```python
from build123d import *

# Parameters (mm, degrees)
SKETCH1_R               = 1.75
BOSS_EXTRUDE3_DEPTH     = 3
SKETCH4_W               = 38.009499712
SKETCH4_H               = 2.5
CUT_EXTRUDE7_DEPTH      = 29.268853886
SKETCH7_W               = 36
SKETCH7_H               = 1
CUT_EXTRUDE8_DEPTH      = 47.877632193
SKETCH9_W               = 39.982004405
SKETCH9_H               = 3.901650926
SKETCH9_W_2             = 38.509499712
SKETCH9_H_2             = 2.8
SKETCH9_W_3             = 37.982004405
SKETCH9_H_3             = 0.55
CUT_EXTRUDE9_DEPTH      = 10
SKETCH10_W              = 40
SKETCH10_H              = 4
SKETCH10_W_2            = 39.982004405
SKETCH10_H_2            = 3.901650926
CUT_EXTRUDE11_DEPTH     = 29.180278565
SKETCH11_W              = 20
SKETCH11_H              = 3.116121774
CUT_EXTRUDE12_DEPTH     = 10
SKETCH12_W              = 2
SKETCH12_H              = 8.5
CUT_EXTRUDE15_DEPTH     = 10
CROQUIS1_W              = 24
CROQUIS1_H              = 4
SALIENTE_EXTRUIR1_DEPTH = 2
CROQUIS2_W              = 40
CROQUIS2_H              = 4
SALIENTE_EXTRUIR2_DEPTH = 4
CORTAR_EXTRUIR2_DEPTH   = 4
SKETCH3_W               = 9
SKETCH3_H               = 3.998143652
CORTAR_EXTRUIR5_DEPTH   = 4


with BuildPart() as part:
    # Sketch1 → Boss-Extrude3 (new body)
    # profile 1 of 2: a face of its own
    with BuildSketch(Plane(origin=(0, 0, 0), x_dir=(1, 0, 0), z_dir=(0, 1, 0))):
        Polygon((-21.59, 18), (-21.59, 0), (0, 0), (21.59, 0), (21.59, 18), (18.04585781, 18), (10.04585781, 18), (10.04585781, 12.616121774), (-9.95414219, 12.616121774), (-9.95414219, 18), (-17.95414219, 18), align=None)
        with Locations(Location((-15, 15, 0), (0, 0, 270))):
            Circle(SKETCH1_R, mode=Mode.SUBTRACT)
        Polygon((18.504745017, 6.25), (0, 6.25), (-18.5, 6.25), (-19.004539265, 6.25), (-19.004539265, 8.75), (-18.5, 8.75), (0.002372509, 8.75), (18.504745017, 8.75), (19.004960447, 8.75), (19.004960447, 6.25), align=None, mode=Mode.SUBTRACT)
        with Locations(Location((15, 15, 0), (0, 0, 270))):
            Circle(SKETCH1_R, mode=Mode.SUBTRACT)
    # profile 2 of 2: a face of its own
    with BuildSketch(Plane(origin=(0, 0, 0), x_dir=(1, 0, 0), z_dir=(0, 1, 0))):
        Polygon((0, 0), (-21.59, 0), (-21.59, -18), (-17.95414219, -18), (-9.95414219, -18), (-9.95414219, -12.616121774), (10.04585781, -12.616121774), (10.04585781, -18), (18.04585781, -18), (21.59, -18), (21.59, 0), align=None)
        with Locations(Location((-15, -15, 0), (0, 0, 270))):
            Circle(SKETCH1_R, mode=Mode.SUBTRACT)
        with Locations(Location((15, -15, 0), (0, 0, 270))):
            Circle(SKETCH1_R, mode=Mode.SUBTRACT)
        Polygon((18.504745017, -6.25), (19.004960447, -6.25), (19.004960447, -8.75), (18.504745017, -8.75), (-18.5, -8.75), (-19.004539265, -8.75), (-19.004539265, -6.25), (-18.5, -6.25), align=None, mode=Mode.SUBTRACT)
    extrude(amount=BOSS_EXTRUDE3_DEPTH)

    # Sketch4 → Cut-Extrude7 (cut, through all)
    # profile 1 of 3: a face of its own
    with BuildSketch(Plane(origin=(0, 3, 0), x_dir=(1, 0, 0), z_dir=(0, 1, 0))):
        Polygon((19.004960447, 6.1), (19.254960447, 6.1), (19.254960447, 8.882786661), (19.254960447, 8.9), (19.004960447, 8.9), (-19.004539265, 8.9), (-19.254539265, 8.9), (-19.254539265, 6.1), (-19.004539265, 6.1), align=None)
        with Locations((0.000210591, 7.5)):
            Rectangle(SKETCH4_W, SKETCH4_H, mode=Mode.SUBTRACT)
    # profile 2 of 3: a face of its own
    with BuildSketch(Plane(origin=(0, 3, 0), x_dir=(1, 0, 0), z_dir=(0, 1, 0))):
        with Locations((0.000210591, 7.5)):
            Rectangle(SKETCH4_W, SKETCH4_H)
    # profile 3 of 3: a face of its own
    with BuildSketch(Plane(origin=(0, 3, 0), x_dir=(1, 0, 0), z_dir=(0, 1, 0))):
        Polygon((-19.254539265, -6.1), (-19.254539265, -8.9), (-19.004539265, -8.9), (19.004960447, -8.9), (19.254960447, -8.9), (19.254960447, -6.1), (19.004960447, -6.1), (-19.004539265, -6.1), align=None)
        with Locations((0.000210591, -7.5)):
            Rectangle(SKETCH4_W, SKETCH4_H, mode=Mode.SUBTRACT)
    extrude(amount=-CUT_EXTRUDE7_DEPTH, mode=Mode.SUBTRACT)

    # Sketch7 → Cut-Extrude8 (cut, through all)
    with BuildSketch(Plane(origin=(21.59, 0, 0), x_dir=(0, 0, -1), z_dir=(1, 0, 0))):
        with Locations((0, 0.5)):
            Rectangle(SKETCH7_W, SKETCH7_H)
    extrude(amount=-CUT_EXTRUDE8_DEPTH, mode=Mode.SUBTRACT)

    # Sketch9 → Cut-Extrude9 (cut)
    # profile 1 of 4: a face of its own
    with BuildSketch(Plane(origin=(0, 3, 0), x_dir=(1, 0, 0), z_dir=(0, 1, 0))):
        with Locations((0.000210592, 7.5)):
            Rectangle(SKETCH9_W, SKETCH9_H)
        with Locations((0.000210591, 7.5)):
            Rectangle(SKETCH9_W_2, SKETCH9_H_2, mode=Mode.SUBTRACT)
    # profile 2 of 4: a face of its own
    with BuildSketch(Plane(origin=(0, 3, 0), x_dir=(1, 0, 0), z_dir=(0, 1, 0))):
        with Locations((0.000210592, -7.5)):
            Rectangle(SKETCH9_W, SKETCH9_H)
        Polygon((-19.254539265, -8.9), (-19.254539265, -6.1), (-18.990791611, -6.1), (-18.990791611, -5.55), (18.991212794, -5.55), (18.991212794, -6.1), (19.254960447, -6.1), (19.254960447, -8.9), (18.991212794, -8.9), (18.991212794, -9.45), (-18.990791611, -9.45), (-18.990791611, -8.9), align=None, mode=Mode.SUBTRACT)
    # profile 3 of 4: a face of its own
    with BuildSketch(Plane(origin=(0, 3, 0), x_dir=(1, 0, 0), z_dir=(0, 1, 0))):
        with Locations((0.000210592, -5.825)):
            Rectangle(SKETCH9_W_3, SKETCH9_H_3)
    # profile 4 of 4: a face of its own
    with BuildSketch(Plane(origin=(0, 3, 0), x_dir=(1, 0, 0), z_dir=(0, 1, 0))):
        with Locations((0.000210592, -9.175)):
            Rectangle(SKETCH9_W_3, SKETCH9_H_3)
    extrude(amount=-CUT_EXTRUDE9_DEPTH, mode=Mode.SUBTRACT)

    # Sketch10 → Cut-Extrude11 (cut, through all)
    # profile 1 of 3: a face of its own
    with BuildSketch(Plane(origin=(0, 3, 0), x_dir=(1, 0, 0), z_dir=(0, 1, 0))):
        with Locations((0.000210591, -7.5)):
            Rectangle(SKETCH10_W, SKETCH10_H)
        with Locations((0.000210592, -7.5)):
            Rectangle(SKETCH10_W_2, SKETCH10_H_2, mode=Mode.SUBTRACT)
    # profile 2 of 3: a face of its own
    with BuildSketch(Plane(origin=(0, 3, 0), x_dir=(1, 0, 0), z_dir=(0, 1, 0))):
        with Locations((0.000210591, 7.5)):
            Rectangle(SKETCH10_W, SKETCH10_H)
        with Locations((0.000210592, 7.5)):
            Rectangle(SKETCH10_W_2, SKETCH10_H_2, mode=Mode.SUBTRACT)
    # profile 3 of 3: a face of its own
    with BuildSketch(Plane(origin=(0, 3, 0), x_dir=(1, 0, 0), z_dir=(0, 1, 0))):
        with Locations((0.000210592, 7.5)):
            Rectangle(SKETCH10_W_2, SKETCH10_H_2)
    extrude(amount=-CUT_EXTRUDE11_DEPTH, mode=Mode.SUBTRACT)

    # Sketch11 → Cut-Extrude12 (cut)
    with BuildSketch(Plane(origin=(0, 3, 0), x_dir=(1, 0, 0), z_dir=(0, 1, 0))):
        with Locations((0.04585781, -11.058060887)):
            Rectangle(SKETCH11_W, SKETCH11_H)
        with Locations((0.04585781, 11.058060887)):
            Rectangle(SKETCH11_W, SKETCH11_H)
    extrude(amount=-CUT_EXTRUDE12_DEPTH, mode=Mode.SUBTRACT)

    # Sketch12 → Cut-Extrude15 (cut)
    with BuildSketch(Plane(origin=(0, 3, 0), x_dir=(1, 0, 0), z_dir=(0, 1, 0))):
        with Locations((-10.95414219, -13.75)):
            Rectangle(SKETCH12_W, SKETCH12_H)
        with Locations((-10.95414219, 13.75)):
            Rectangle(SKETCH12_W, SKETCH12_H)
        with Locations((11.04585781, 13.75)):
            Rectangle(SKETCH12_W, SKETCH12_H)
        Polygon((10.04585781, -9.65592739), (10.04585781, -18), (12.04585781, -18), (12.04585781, -9.65592739), (12.04585781, -9.5), (10.04585781, -9.5), align=None)
    extrude(amount=-CUT_EXTRUDE15_DEPTH, mode=Mode.SUBTRACT)

    # Croquis1 → Saliente-Extruir1 (add)
    with BuildSketch(Plane(origin=(0, 3, 0), x_dir=(1, 0, 0), z_dir=(0, 1, 0))):
        with Locations((0.04585781, -11.5)):
            Rectangle(CROQUIS1_W, CROQUIS1_H)
        with Locations((0.04585781, 11.5)):
            Rectangle(CROQUIS1_W, CROQUIS1_H)
    extrude(amount=-SALIENTE_EXTRUIR1_DEPTH)

    # Croquis2 → Saliente-Extruir2 (add)
    with BuildSketch(Plane(origin=(0, 3, 0), x_dir=(1, 0, 0), z_dir=(0, 1, 0))):
        Polygon((21.59, 9.27), (21.59, 12.25), (-21.59, 12.25), (-21.59, 9.27), (-21.59, -9.27), (-21.59, -12.25), (21.59, -12.25), (21.59, -9.27), align=None)
        with Locations((0.000210591, -7.5)):
            Rectangle(CROQUIS2_W, CROQUIS2_H, mode=Mode.SUBTRACT)
        with Locations((0.000210591, 7.5)):
            Rectangle(CROQUIS2_W, CROQUIS2_H, mode=Mode.SUBTRACT)
    extrude(amount=SALIENTE_EXTRUIR2_DEPTH)

    # Croquis4 → Cortar-Extruir2 (cut)
    with BuildSketch(Plane.XZ.offset(-1)):
        Polygon((-21.59, -9.5), (-21.59, 9.5), (-19.999789409, 9.5), (-19.999789409, 5.5), (20.000210591, 5.5), (20.000210591, 9.5), (21.59, 9.5), (21.59, -9.5), (20.000210591, -9.5), (20.000210591, -5.5), (-19.999789409, -5.5), (-19.999789409, -9.5), align=None)
    extrude(amount=-CORTAR_EXTRUIR2_DEPTH, mode=Mode.SUBTRACT)

    # Sketch3 → Cortar-Extruir5 (cut)
    with BuildSketch(Plane(origin=(0, 3, 0), x_dir=(1, 0, 0), z_dir=(0, 1, 0))):
        Polygon((-1.911780511, -2), (-1.911780511, 0), (-3.40804733, 0), (-3.911780511, 0), (-3.911780511, -0.084828213), (-3.911780511, -2), align=None)
        Polygon((-3.40804733, 0), (-1.911780511, 0), (-1.911780511, 2), (-3.911780511, 2), (-3.911780511, 0), align=None)
        Polygon((12.59, 0.000697543), (12.59, 0), (21.59, 0), (21.59, 3.999538738), (12.59, 3.999538738), align=None)
        with Locations((17.09, -1.999071826)):
            Rectangle(SKETCH3_W, SKETCH3_H)
        Polygon((-16.59, -3.75), (-16.59, 0), (-16.59, 3.75), (-21.59, 3.75), (-21.59, 0), (-21.59, -3.75), align=None)
    extrude(amount=CORTAR_EXTRUIR5_DEPTH, mode=Mode.SUBTRACT)


solid = part.part
```
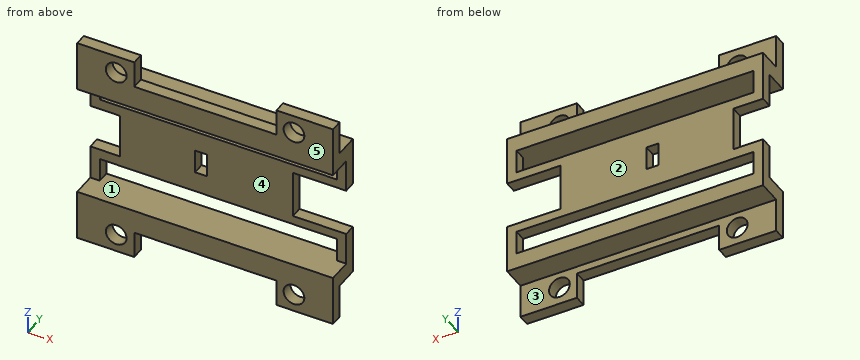
The listing builds one solid part. Answer for the finished solid, in the listing's coordinates (mm). Face numbers are marked on the shaded views. A direction names the side the tool comes from. Give positions to 0.01 mm unless a question says otherwise; leave off trailing zeros. Order: outer loops, then holes, each group sorted by start corner. A loop starts at its lowest first (then second) coordinate and runs counter-clockwise, first axis right, second up.
1) For the marked faces 3, 4 and 5, determine the directions among +Z, -Z, +X, -X, +Y, -Y from which every point of the face is accessible in a straight line to the end or side of a thin tool.
Reported:
face 3: -Z, +X, -X, +Y
face 4: +X, -X, -Y
face 5: +Z, -Z, +X, -X, -Y
2) Determine the mould class of the marked faces 1 and 2 for opening direction X: pulls with the +X half, pulls with the -X half, needs draft (parallel to the pull), parting line crosses it, or undercut.
Reported:
face 1: undercut
face 2: needs draft
3) Find section D-D on z = -15. Write down the section's boundary in (x, y), then the cut area to 3 significant figures.
Reported:
outline: (-21.59, 1) - (-16.75, 1) - (-16.75, 3) - (-21.59, 3) - close; (-13.25, 1) - (-11.95, 1) - (-11.95, 3) - (-13.25, 3) - close; (12.05, 1) - (13.25, 1) - (13.25, 3) - (12.05, 3) - close; (16.75, 1) - (21.59, 1) - (21.59, 3) - (16.75, 3) - close
area: 24.4 mm2
4) Find section B-B on x = 15. Write down the section's boundary in (y, z), then the cut area to 3 significant figures.
Reported:
outline: (1, -18) - (3, -18) - (3, -16.75) - (1, -16.75) - close; (1, -13.25) - (3, -13.25) - (3, -12.25) - (7, -12.25) - (7, -9.5) - (1, -9.5) - close; (1, 9.5) - (7, 9.5) - (7, 12.25) - (3, 12.25) - (3, 13.25) - (1, 13.25) - close; (1, 16.75) - (3, 16.75) - (3, 18) - (1, 18) - close; (5, -5.5) - (7, -5.5) - (7, -4) - (5, -4) - close; (5, 4) - (7, 4) - (7, 5.5) - (5, 5.5) - close
area: 48.0 mm2
5) Find section C-C on x = -15. Write down the section's boundary in (y, z).
Reported:
outline: (1, -18) - (3, -18) - (3, -16.75) - (1, -16.75) - close; (1, -13.25) - (3, -13.25) - (3, -12.25) - (7, -12.25) - (7, -9.5) - (1, -9.5) - close; (1, 9.5) - (7, 9.5) - (7, 12.25) - (3, 12.25) - (3, 13.25) - (1, 13.25) - close; (1, 16.75) - (3, 16.75) - (3, 18) - (1, 18) - close; (5, -5.5) - (7, -5.5) - (7, 5.5) - (5, 5.5) - close
6) Consider line 1 along Z through (x, y) = (-9, 6.3); line 2 along X through (y, z) = (1.7, -15); line 3 along Z through (x, y) = (15, 2.05). Determine where each line is inside the solid, lowest interval first.
Reported:
line 1: z = -12.25 to -9.5, -5.5 to 5.5, 9.5 to 12.25
line 2: x = -21.59 to -16.75, -13.25 to -11.95, 12.05 to 13.25, 16.75 to 21.59
line 3: z = -18 to -16.75, -13.25 to -9.5, 9.5 to 13.25, 16.75 to 18
7) Find section A-A on y = 2. Write down the section's boundary in (x, z).
Reported:
outline: (-21.59, -18) - (-11.95, -18) - (-11.95, -13.5) - (12.05, -13.5) - (12.05, -18) - (21.59, -18) - (21.59, -9.5) - (-21.59, -9.5) - close; (-21.59, 9.5) - (21.59, 9.5) - (21.59, 18) - (12.05, 18) - (12.05, 13.5) - (-11.95, 13.5) - (-11.95, 18) - (-21.59, 18) - close; hole circle Ø3.5 at (-15, -15); hole circle Ø3.5 at (-15, 15); hole circle Ø3.5 at (15, -15); hole circle Ø3.5 at (15, 15)
8) Given P1, Ø1.6, axis at y = 5.5, z = -1.5, coming from the -X side; P2, Ø4, axis at x = 10.5, z = 14, coming from the -Y side; P3, Ø6, axis at x = 3.5, z = 0, coming from the -Y side; P4, Ø0.6, axis at x = -3, y = 6, coming from the +Z side, each flat-ended and moving along its own axis, determine where each tip first touches the part or whether it passes through.
Reported:
P1: stops at x = -16.59
P2: stops at y = 1
P3: stops at y = 5
P4: stops at z = 12.25
